Input: part model. Units: mm. Frame: model coordinates. Face numbers are marked on the shaded views. A direction names the side the tool comes from. Coordinates: 2 decimals unless noted, no trailing zeros. Order: outer loops, then holes, each group sorted by start corner. A loop starts at its lowest first (then second) coordinate and runs counter-clockwise, first axis right, second up. Notation, with made-up numbers: M -30.5,65 L -18.5,65 A14 cw -18.5,80 Z; hole C -30.75,30.25 d2. An arc over 180 degrees is marked long. Answer in a Markdown table with one row per item.
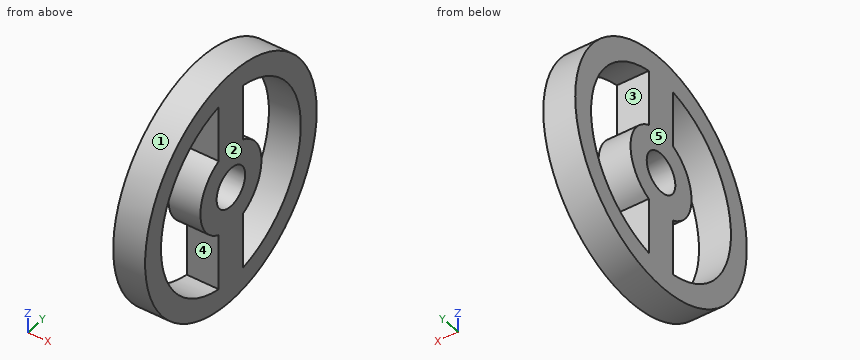
from build123d import *

# Parameters (mm, degrees)
F0_R     = 19.05
F0_R_2   = 3.175
F1_DEPTH = 5.08


with BuildPart() as f1:
    # F0 (on Right) → F1 (new body)
    with BuildSketch(Plane.YZ):
        Circle(F0_R)
        with BuildLine():
            ThreePointArc((-2.712303, -15.287515), (-15.526259, 0), (-2.712303, 15.287515))
            Line((-2.712303, 15.287515), (-2.712303, 6.20612))
            ThreePointArc((-2.712303, 6.20612), (-6.772925, 0), (-2.712303, -6.20612))
            Line((-2.712303, -6.20612), (-2.712303, -15.287515))
        make_face(mode=Mode.SUBTRACT)
        Circle(F0_R_2, mode=Mode.SUBTRACT)
        with BuildLine():
            Line((2.712303, 6.20612), (2.712303, 15.287515))
            ThreePointArc((2.712303, 15.287515), (15.526259, 0.002746), (2.717711, -15.286555))
            Line((2.717711, -15.286555), (2.717711, -6.203754))
            ThreePointArc((2.717711, -6.203754), (6.772924, 0.002951), (2.712303, 6.20612))
        make_face(mode=Mode.SUBTRACT)
    extrude(amount=F1_DEPTH)


solid = f1.part
1) Cut plane D-D, the plane y = 5. Output: boundary loops of the cut face in (x, z).
Resolved:
| item | result |
|---|---|
| outline | M 0,-18.38 L 5.08,-18.38 L 5.08,-14.7 L 0,-14.7 Z; M 0,-4.57 L 5.08,-4.57 L 5.08,4.57 L 0,4.57 Z; M 0,14.7 L 5.08,14.7 L 5.08,18.38 L 0,18.38 Z |
2) Cut plane B-B, the plane y = 0. Output: boundary loops of the cut face in (x, z) (3 decimals).
Resolved:
| item | result |
|---|---|
| outline | M 0,-19.05 L 5.08,-19.05 L 5.08,-3.175 L 0,-3.175 Z; M 0,3.175 L 5.08,3.175 L 5.08,19.05 L 0,19.05 Z |
3) Contact query for flat-ended pins moving along their axis: pin 1 (2.5 mm diameter, centred on x = 2, z = 11, fed in from -Y); pin 2 (1.5 mm diameter, centred on x = 1, z = 15, fed in from -Y); pin 3 (6 mm diameter, centred on y = 7, z = -8, fed in from -X); pin 4 (2.5 mm diameter, centred on x = 2.5, z = -9.5, fed in from -Y). Output: stop coordinate, or through.
Resolved:
| item | result |
|---|---|
| pin 1 | stops at y = -16.37 |
| pin 2 | stops at y = -12.64 |
| pin 3 | passes through |
| pin 4 | stops at y = -17.17 |
4) Mould query, pull axis Z, two halves, no side actions, for the marked faces 1, 2 and 3. Classes: +Z half, -Z half, draft (parallel to the pull), parting line (faces both ways), or undercut.
Resolved:
| item | result |
|---|---|
| face 1 | parting line |
| face 2 | draft |
| face 3 | undercut |
5) Cut plane A-A, the plane z = 0. Output: boundary loops of the cut face in (x, y) (3 decimals).
Resolved:
| item | result |
|---|---|
| outline | M 0,-19.05 L 5.08,-19.05 L 5.08,-15.526 L 0,-15.526 Z; M 0,-6.773 L 5.08,-6.773 L 5.08,-3.175 L 0,-3.175 Z; M 0,3.175 L 5.08,3.175 L 5.08,6.773 L 0,6.773 Z; M 0,15.526 L 5.08,15.526 L 5.08,19.05 L 0,19.05 Z |
6) Material intervals for probe 1 along Z at (x, y) = (3.15, 0) (3 decimals); probe 2 along Y at (x, z) = (1.25, 8); probe 3 along Y at (x, z) = (4.7, 3.5), sorted ascending.
Resolved:
| item | result |
|---|---|
| probe 1 | z = -19.05 to -3.175, 3.175 to 19.05 |
| probe 2 | y = -17.29 to -13.31, -2.71 to 2.71, 13.31 to 17.29 |
| probe 3 | y = -18.73 to -15.13, -5.8 to 5.8, 15.13 to 18.73 |
7) Cut plane C-C, the plane x = 3.4. Output: boundary loops of the cut face in (y, z) (3 decimals).
Resolved:
| item | result |
|---|---|
| outline | C 0,0 d38.1; hole C 0,0 d6.35; hole M -2.712,-15.288 L -2.712,-6.206 A6.773 cw -2.712,6.206 L -2.712,15.288 A15.526 ccw Z; hole M 2.712,6.206 A6.773 cw 2.718,-6.204 L 2.718,-15.287 A15.526 ccw 2.712,15.288 Z |
8) Reachability of the marked faces 4 and 5 from +Z, -Z, +X, -X, +Y, -Y: full face, straight path, thin tool, end or side. Return the list, or none.
Resolved:
| item | result |
|---|---|
| face 4 | +X, -X |
| face 5 | +Z, -Z, -X, +Y, -Y |
